```python
from build123d import *

# Parameters (mm, degrees)
F1_DEPTH = 3
F2_W     = 0.15
F2_H     = 3
F3_DEPTH = 1.5
F4_SIZE  = 1
F5_R     = 1


with BuildPart() as f1:
    # F0 (on Top) → F1 (new body)
    with BuildSketch(Plane.XY):
        Polygon((2, 22), (-4, 16), (-4, 0), (0, 0), (0, 13.4), (2, 15.4), (4, 15.4), (4, 22), align=None)
    extrude(amount=F1_DEPTH)

    # F2 (on face) → F3 (join)
    with BuildSketch(Plane.YZ.offset(4)):
        with Locations((15.325, 1.5)):
            Rectangle(F2_W, F2_H)
        with Locations((22.075, 1.5)):
            Rectangle(F2_W, F2_H)
    extrude(amount=-F3_DEPTH)

    # F4
    f4_edges = [f1.edges().sort_by_distance(p)[0] for p in [
        (4, 15.25, 1.5),
        (4, 22.15, 1.5),
    ]]
    chamfer(f4_edges, length=F4_SIZE)

    # F5
    f5_edges = [f1.edges().sort_by_distance(p)[0] for p in [
        (0, 0, 1.5),
        (-4, 0, 1.5),
    ]]
    fillet(f5_edges, radius=F5_R)


solid = f1.part
```
Geometry check sheet. Reference: the model listing, model coordinates, mm. A direction names the side the tool comes from. Coordinates: 2 decimals unless noted, no trailing zeros. Loops run counter-clockwise (first coordinate to the right, second up) from the corner with the lowest first, then second, coordinate; pieces in that order, holes last.
Item 1: Sectioned sample at C-C, the plane y = 9.25. Record the boundary of the cut face in (x, z).
Item 2: Access from +Z, -Z, +X, -X, +Y, -Y to the whole of each face (thin tool, end or side, straight path). Record for faces 1 (the face through (-1, 11, 0)), 2 (the face through (0, 7, 1)).
Item 3: Go/stop test with a flat-tipped pin: pin 1 Ø1.5 at (x, z) = (-1, 0.5) entering from +Y. Record where the tip stops, or that it passes through.
Item 4: Thickness scan on line 1 (X direction, y = 8.75, z = 1.7); line 2 (X direction, y = 17, z = 0.6); line 3 (Y direction, x = 1.5, z = 0.95). Record the ranges inside material, lowest first.
Item 5: Sectioned sample at B-B, the plane x = -2.75. Record the boundary of the cut face in (y, z), then the cut area to 4 significant figures.
Item 6: Sectioned sample at A-A, the plane z = 1.05. Record the boundary of the cut face in (x, y).
Check result:
1. outline: (-4, 0) - (0, 0) - (0, 3) - (-4, 3) - close
2. face 1: -Z, +X, -X, +Y, -Y
2. face 2: +Z, -Z, +X, -Y
3. pin 1: stops at y = 19.75
4. line 1: x = -4 to 0
4. line 2: x = -3 to 4
4. line 3: y = 14.9 to 21.5
5. outline: (0, 0) - (17.25, 0) - (17.25, 3) - (0, 3) - close
5. area: 51.75 mm2
6. outline: (-4, 1) arc R1 ccw to (-3, 0) - (-1, 0) arc R1 ccw to (0, 1) - (0, 13.4) - (2, 15.4) - (2.5, 15.4) - (2.5, 15.25) - (3, 15.25) - (4, 16.25) - (4, 21.15) - (3, 22.15) - (2.5, 22.15) - (2.5, 22) - (2, 22) - (-4, 16) - close
